```python
from build123d import *

# Parameters (mm, degrees)
SKETCH1_W           = 69.85
SKETCH1_H           = 76.2
SKETCH1_R           = 2.38125
BOSS_EXTRUDE1_DEPTH = 6.35
FILLET1_R           = 2.54


with BuildPart() as part:
    # Sketch1 → Boss-Extrude1 (new body)
    with BuildSketch(Plane(origin=(0, 0, 0), x_dir=(1, 0, 0), z_dir=(0, 1, 0))):
        Rectangle(SKETCH1_W, SKETCH1_H)
        with Locations(Location((22.225, 0, 0), (0, 0, 270))):
            Circle(SKETCH1_R, mode=Mode.SUBTRACT)
        with Locations(Location((22.225, -25.4, 0), (0, 0, 270))):
            Circle(SKETCH1_R, mode=Mode.SUBTRACT)
        with Locations(Location((22.225, 25.4, 0), (0, 0, 270))):
            Circle(SKETCH1_R, mode=Mode.SUBTRACT)
        with Locations(Location((-28.575, -25.4, 0), (0, 0, 270))):
            Circle(SKETCH1_R, mode=Mode.SUBTRACT)
        with Locations(Location((-28.575, 19.05, 0), (0, 0, 270))):
            Circle(SKETCH1_R, mode=Mode.SUBTRACT)
        with Locations(Location((-28.575, 6.35, 0), (0, 0, 270))):
            Circle(SKETCH1_R, mode=Mode.SUBTRACT)
        with Locations(Location((-3.175, -25.4, 0), (0, 0, 270))):
            Circle(SKETCH1_R, mode=Mode.SUBTRACT)
        with Locations(Location((-3.175, 19.05, 0), (0, 0, 270))):
            Circle(SKETCH1_R, mode=Mode.SUBTRACT)
        with Locations(Location((-3.175, 6.35, 0), (0, 0, 270))):
            Circle(SKETCH1_R, mode=Mode.SUBTRACT)
    extrude(amount=BOSS_EXTRUDE1_DEPTH)

    # Fillet1
    fillet1_edges = [part.edges().sort_by_distance(p)[0] for p in [
        (-34.925, 3.175, 38.1),
        (-34.925, 3.175, -38.1),
    ]]
    fillet(fillet1_edges, radius=FILLET1_R)


solid = part.part
```
Part model, mm, in its own coordinate system. Give positions to 0.01 mm unless a question says otherwise; leave off trailing zeros. Write each loop counter-clockwise with the first axis right and the second up, starting at its lowest first coordinate (ties: lowest second). Pieces come first, ordered by that corner, then holes. Notation, with made-up numbers: (89.5, 67) -> (126.5, 67) arc R10 cw to (126.5, 74) -> close; hole circle Ø7 at (65.5, 85). An arc over 180 degrees is marked (long way). Put each result on its own line as item: value. Start each with the question number.
Item 1: Wall check: L1, parallel to X at y = 5, z = -6.35 (3 decimals); L2, parallel to X at y = 3.5, z = -25.4 (3 decimals); L3, parallel to Z at x = -29, y = 6. Give the ranges that are in metal, low to high. Write a range as [from, to].
Item 2: Pin check, flat tip, straight feed: pin 1 Ø3 at (x, z) = (-28.575, -19.05) entering from +Y. Stop position of the tip, or through.
Item 3: Cut at A-A (z = -25.4). List the corners of the cut face in (x, y) (3 decimals).
Item 4: Cut at B-B (z = 25.4). List the corners of the cut face in (x, y) (3 decimals).
Item 5: Cut at C-C (x = -2). List the corners of the cut face in (y, z), then the cut area to 3 significant figures.
Item 6: Cut at D-D (y = 5). State how many separate pieces and enclosed holes the cut face has, then the cut area to 3 significant figures.
Item 7: Pull direction X, two halves, no side cores. Call faces 1 (the face through (-34.201, 3.219, 37.336)), 2 (the face through (1, 3, -38.1)), 3 (the face through (-3.07, 3.13, -21.43)), 4 (the face through (-30.688, 3.131, -5.251)): pulls with the +X half, pulls with the -X half, needs draft (parallel to the pull), parting line crosses it, or undercut.
Answer list:
1. L1: x = [-34.925, -30.956], [-26.194, -5.556], [-0.794, 34.925]
1. L2: x = [-34.925, 19.844], [24.606, 34.925]
1. L3: z = [-38.1, -21.39], [-16.71, -8.69], [-4.01, 23.06], [27.74, 38.1]
2. pin 1: passes through
3. outline: (-34.925, 0) -> (19.844, 0) -> (19.844, 6.35) -> (-34.925, 6.35) -> close; (24.606, 0) -> (34.925, 0) -> (34.925, 6.35) -> (24.606, 6.35) -> close
4. outline: (-34.925, 0) -> (-30.956, 0) -> (-30.956, 6.35) -> (-34.925, 6.35) -> close; (-26.194, 0) -> (-5.556, 0) -> (-5.556, 6.35) -> (-26.194, 6.35) -> close; (-0.794, 0) -> (19.844, 0) -> (19.844, 6.35) -> (-0.794, 6.35) -> close; (24.606, 0) -> (34.925, 0) -> (34.925, 6.35) -> (24.606, 6.35) -> close
5. outline: (0, -38.1) -> (6.35, -38.1) -> (6.35, -21.12) -> (0, -21.12) -> close; (0, -16.98) -> (6.35, -16.98) -> (6.35, -8.42) -> (0, -8.42) -> close; (0, -4.28) -> (6.35, -4.28) -> (6.35, 23.33) -> (0, 23.33) -> close; (0, 27.47) -> (6.35, 27.47) -> (6.35, 38.1) -> (0, 38.1) -> close
5. area: 405 mm2
6. separate pieces: 1
6. enclosed holes: 9
6. area: 5,160 mm2
7. face 1: pulls with the -X half
7. face 2: needs draft
7. face 3: undercut
7. face 4: undercut
